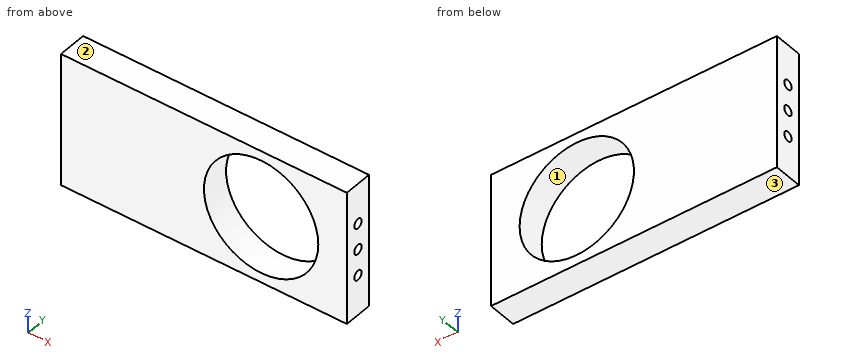
```python
from build123d import *

# Parameters (mm, degrees)
SKETCH1_W           = 190.5
SKETCH1_H           = 88.9
SKETCH1_R           = 38.1
BOSS_EXTRUDE1_DEPTH = 9.525
SKETCH2_R           = 3.175
CUT_EXTRUDE1_DEPTH  = 12.7


with BuildPart() as part:
    # Sketch1 → Boss-Extrude1 (new body, symmetric)
    with BuildSketch(Plane(origin=(0, 0, 0), x_dir=(1, 0, 0), z_dir=(0, 1, 0))):
        Rectangle(SKETCH1_W, SKETCH1_H)
        with Locations((38.1, 0)):
            Circle(SKETCH1_R, mode=Mode.SUBTRACT)
    extrude(amount=BOSS_EXTRUDE1_DEPTH, both=True)

    # Sketch2 → Cut-Extrude1 (cut)
    with BuildSketch(Plane(origin=(95.25, 0, 0), x_dir=(0, 0, -1), z_dir=(1, 0, 0))):
        Circle(SKETCH2_R)
        with Locations((17.526, 0)):
            Circle(SKETCH2_R)
        with Locations((-17.4625, 0)):
            Circle(SKETCH2_R)
    cut_extrude1 = extrude(amount=-CUT_EXTRUDE1_DEPTH, mode=Mode.SUBTRACT)

    # Mirror1: Cut-Extrude1 across plane
    add(cut_extrude1.mirror(Plane(origin=(0, 0, 0), x_dir=(0, 0, 1), z_dir=(1, 0, 0))), mode=Mode.SUBTRACT)


solid = part.part
```
Design review of the part built by this model. Coordinates are the model's own, in mm. Face numbers are marked on the shaded views. Round coordinates to 2 decimals unless told otherwise and drop trailing zeros. Write each loop counter-clockwise with the first axis right and the second up, starting at its lowest first coordinate (ties: lowest second). Pieces come first, ordered by that corner, then holes.
Item 1: We need section C-C on y = -7.75. Write out the cut boundary in (x, z).
Item 2: Clearance check with flat-ended pins moving along their axes: pin 1 Ø1.9 at (y, z) = (1.5, 16) entering from +X; pin 2 Ø1.9 at (y, z) = (-1.5, -16) entering from -X. State where each tip first meets the part, or that it passes through.
Item 3: The part is to be moulded in two halves that separate along Z. For the marked faces 1, 2 and 3, say which applies: +Z half, -Z half, draft (parallel to the pull), parting line (faces both ways), or undercut.
Item 4: We need section B-B on z = 0. Write out the cut boundary in (x, y) (3 decimals), and give its area (3 significant figures).
Item 5: For probe 1 along X at (y, z) = (5.25, 0); probe 2 along Y at (x, z) = (86.75, 0) (3 decimals); probe 3 along Z at (x, y) = (27.5, -6), list the stretches that pass through material, from the lowest coordinate up.
Item 6: We need section A-A on x = 38.1. Write out the cut boundary in (y, z) (3 decimals).
Returned:
1. outline: (-95.25, -44.45) - (95.25, -44.45) - (95.25, 44.45) - (-95.25, 44.45) - close; hole circle Ø76.2 at (38.1, 0)
2. pin 1: stops at x = 82.55
2. pin 2: stops at x = -82.55
3. face 1: undercut
3. face 2: +Z half
3. face 3: -Z half
4. outline: (-95.25, -9.525) - (0, -9.525) - (0, 9.525) - (-95.25, 9.525) - (-95.25, 3.175) - (-82.55, 3.175) - (-82.55, -3.175) - (-95.25, -3.175) - close; (76.2, -9.525) - (95.25, -9.525) - (95.25, -3.175) - (82.55, -3.175) - (82.55, 3.175) - (95.25, 3.175) - (95.25, 9.525) - (76.2, 9.525) - close
4. area: 2,020 mm2
5. probe 1: x = -95.25 to 0, 76.2 to 95.25
5. probe 2: y = -9.525 to -3.175, 3.175 to 9.525
5. probe 3: z = -44.45 to -36.6, 36.6 to 44.45
6. outline: (-9.525, -44.45) - (9.525, -44.45) - (9.525, -38.1) - (-9.525, -38.1) - close; (-9.525, 38.1) - (9.525, 38.1) - (9.525, 44.45) - (-9.525, 44.45) - close
